Job drawing, mm, ordinate dimensions from the low corner. One solid piece. A direction names the side the tool comes from. Round coordinates to 2 decimals unless told otherwise and drop trailing zeros. Loops run counter-clockwise (first coordinate to the right, second up) from the corner with the lowest first, then second, coordinate; pieces in that order, holes last. Notation, with made-up numbers: M 19.5,44.25 L 69.5,44.25 A22 cw 69.5,81.25 Z; hole C -3.5,-27.75 d1. An arc over 180 degrees is marked long. One line per item, written item: value.
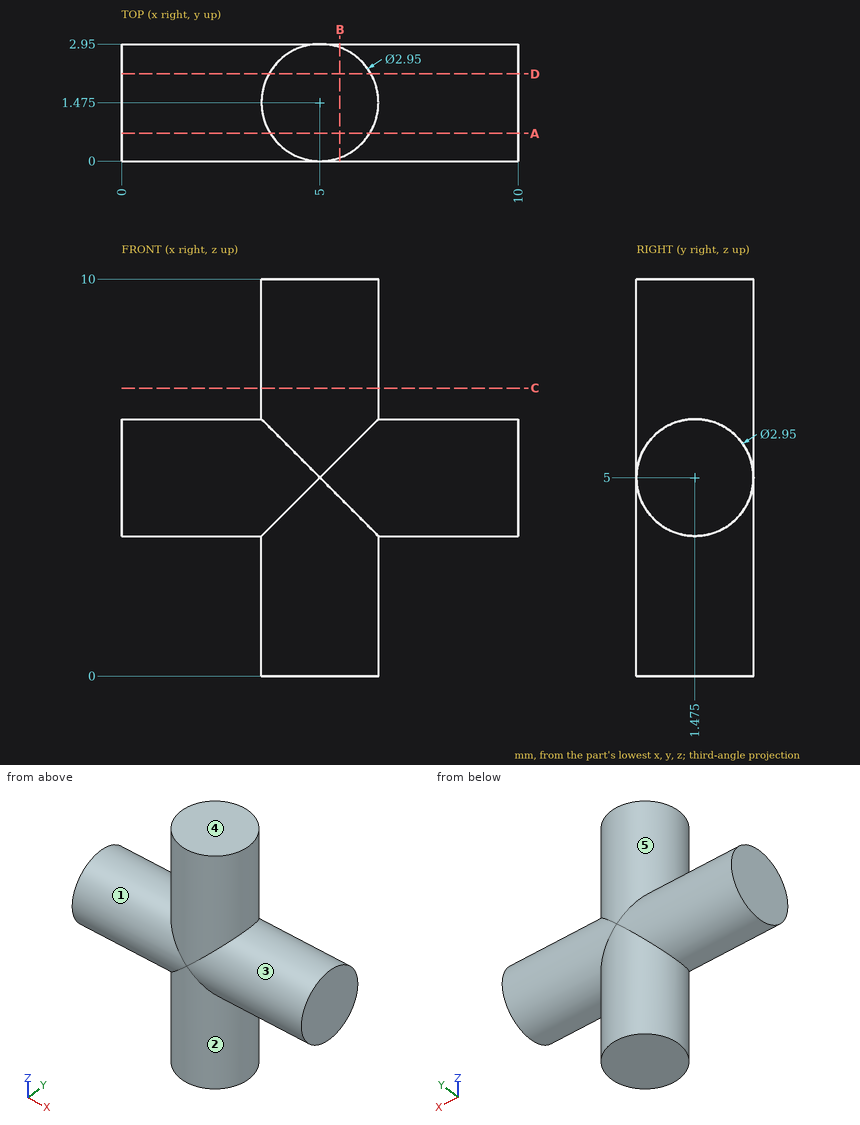
Item 1: Slice it at C-C, the plane z = 7.25. Give the cut face in (x, y) (3 decimals), and give its area (3 significant figures).
Check values:
outline: C 5,1.475 d2.95
area: 6.83 mm2
Item 2: Wall check: line 1 along X through (y, z) = (1.4, 1.5); line 2 along Z through (x, y) = (7, 2.1). Give the ranges that are in metal, low to high.
Check values:
line 1: x = 3.53 to 6.47
line 2: z = 3.66 to 6.34
Item 3: Drop a flat-ended pin along its axis: P1, Ø1.5, axis at x = 2, y = 2.5, coming from the -Z side. Give the stop position or say it passes through.
Check values:
P1: stops at z = 3.55
Item 4: Slice it at A-A, the plane y = 0.7. Give the cut face in (x, z) (3 decimals), and give its area (3 significant figures).
Check values:
outline: M 0,3.745 L 3.745,3.745 L 3.745,0 L 6.255,0 L 6.255,3.745 L 10,3.745 L 10,6.255 L 6.255,6.255 L 6.255,10 L 3.745,10 L 3.745,6.255 L 0,6.255 Z
area: 43.9 mm2
Item 5: Which spindle directions (+Z, -Z, +X, -X, +Y, -Y) get a long thin tool onto all of the face, cutting with end or side? Do the marked faces 1, 2, 3, 4 and 5. Say none if no direction does.
Check values:
face 1: -X
face 2: -Z
face 3: +X
face 4: +Z, +X, -X, +Y, -Y
face 5: +Z
Item 6: Slice it at B-B, the plane x = 5.5. Give the cut face in (y, z) (3 decimals).
Check values:
outline: M 0.087,0 L 2.863,0 L 2.863,4.5 A1.475 ccw 2.863,5.5 L 2.863,10 L 0.087,10 L 0.087,5.5 A1.475 ccw 0.087,4.5 Z
Item 7: Slice it at D-D, the plane y = 2.2. Give the cut face in (x, z).
Check values:
outline: M 0,3.72 L 3.72,3.72 L 3.72,0 L 6.28,0 L 6.28,3.72 L 10,3.72 L 10,6.28 L 6.28,6.28 L 6.28,10 L 3.72,10 L 3.72,6.28 L 0,6.28 Z
